Geometry check sheet. Reference: drawing and pictorial views, mm from the part's lowest x, y, z. Give positions to 0.01 mm unless a question says otherwise; leave off trailing zeros. Loops run counter-clockwise (first coordinate to the right, second up) from the corner with the lowest first, then second, coordinate; pieces in that order, holes last. Notation, with made-up numbers: M 13.25,4.5 L 21.25,4.5 A20 cw 21.25,38.5 Z; hole C 8.5,-40 d1. An arc over 180 degrees is marked long. Put each result on its own line as item: value. Start each with the question number.
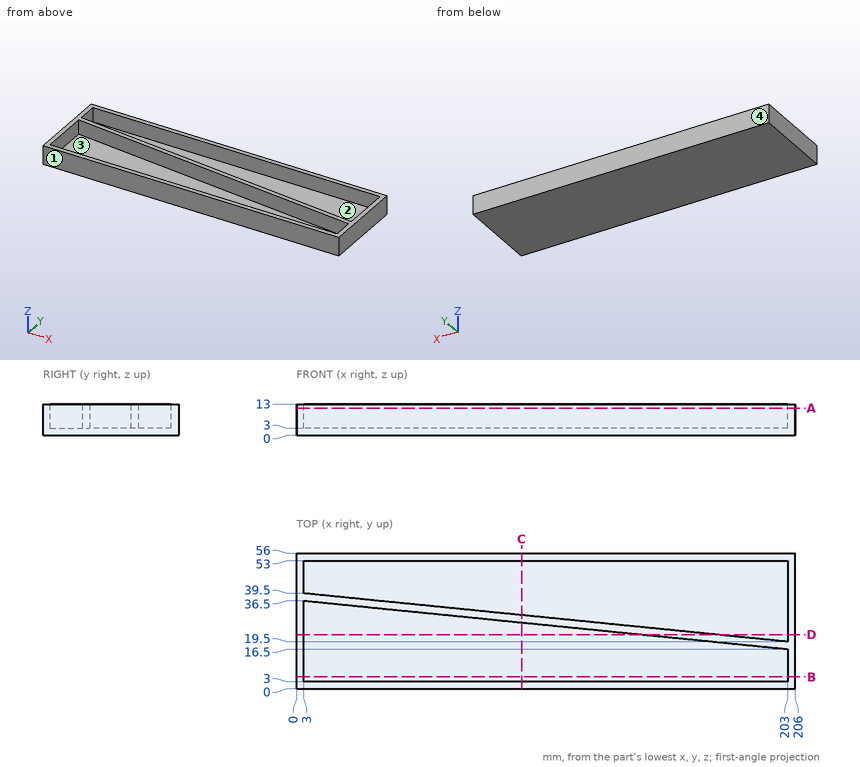
Q1. Section check D-D, the plane y = 22.5. Record the cut outline in (x, z).
Q2. Section check A-A, the plane z = 11.25. Record the cut outline in (x, y).
Q3. Depth check by flat-ended pin: P1, Ø6, axis at y = 20, z = 2.5, coming from the -X side. Enter the tip coordinate at first touch or a pass-through.
Q4. Section check C-C, the plane x = 93. Record the cut outline in (y, z), then the cut area to 3 significant figures.
Q5. Section check B-B, the plane y = 5. Record the cut outline in (x, z).
Q6. Mould release check, pull along Y, two halves, no side actions. Record for the marked faces 1, 2, 3 and 4: pulls with the +Y half, pulls with the -Y half, needs draft (parallel to the pull), parting line crosses it, or undercut.
Q7. Thickness scan on line 1 along Y through (x, z) = (178, 10.5); line 2 along Y through (x, z) = (113, 10.75); line 3 along X through (y, z) = (11, 8.5). Record the ranges inside material, lowest first. Write a range as [from, to].
Found:
1. outline: M 0,0 L 206,0 L 206,13 L 203,13 L 203,3 L 173,3 L 173,13 L 143,13 L 143,3 L 3,3 L 3,13 L 0,13 Z
2. outline: M 0,0 L 206,0 L 206,56 L 0,56 Z; hole M 3,3 L 203,3 L 203,16.5 L 3,36.5 Z; hole M 3,39.5 L 203,19.5 L 203,53 L 3,53 Z
3. P1: stops at x = 0
4. outline: M 0,0 L 56,0 L 56,13 L 53,13 L 53,3 L 30.5,3 L 30.5,13 L 27.5,13 L 27.5,3 L 3,3 L 3,13 L 0,13 Z
4. area: 258 mm^2
5. outline: M 0,0 L 206,0 L 206,13 L 203,13 L 203,3 L 3,3 L 3,13 L 0,13 Z
6. face 1: pulls with the -Y half
6. face 2: undercut
6. face 3: undercut
6. face 4: pulls with the +Y half
7. line 1: y = [0, 3], [19, 22], [53, 56]
7. line 2: y = [0, 3], [25.5, 28.5], [53, 56]
7. line 3: x = [0, 3], [203, 206]
